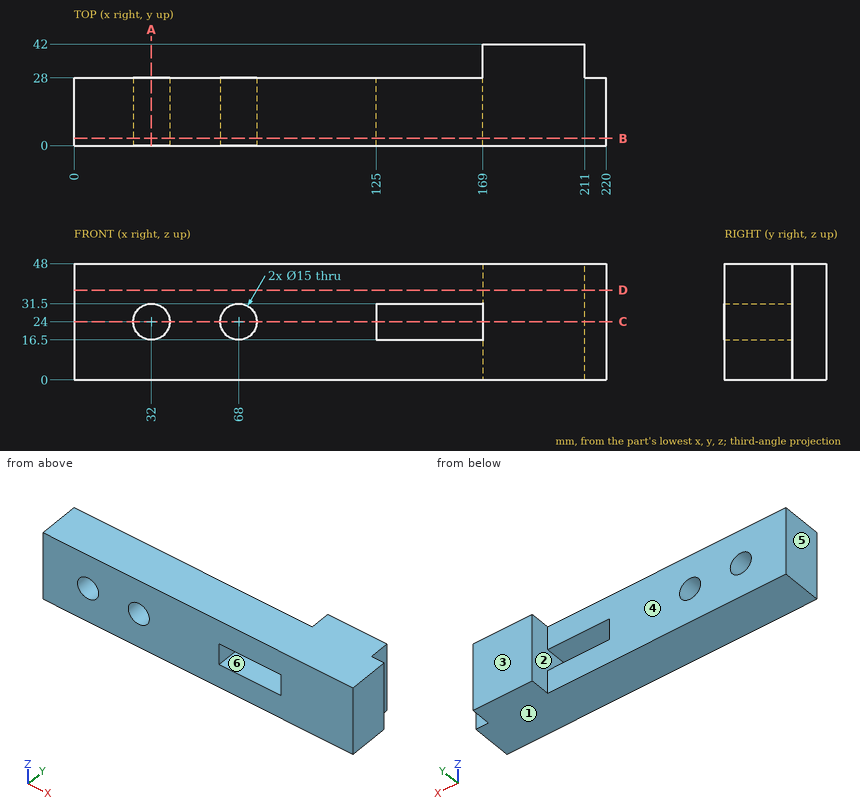
Source: three-view drawing plus pictorial views. Frame: mm from the lowest corner of the part. A direction names the side the tool comes from. Round coordinates to 2 decimals unless told otherwise and drop trailing zeros. Loops run counter-clockwise (first coordinate to the right, second up) from the corner with the lowest first, then second, coordinate; pieces in that order, holes last.
Item 1: Section B-B, the plane y = 3. Output: boundary loops of the cut face in (x, z).
Checked values:
outline: (0, 0) - (220, 0) - (220, 48) - (0, 48) - close; hole circle Ø15 at (32, 24); hole circle Ø15 at (68, 24); hole (125, 16.5) - (169, 16.5) - (169, 31.5) - (125, 31.5) - close
Item 2: Contact query for flat-ended pins moving along their axis: P1, Ø4.5, axis at x = 217, z = 14, coming from the +Y side; P2, Ø8, axis at y = 34.5, z = 12.5, coming from the -X side. Output: stop coordinate, or through.
Checked values:
P1: stops at y = 28
P2: stops at x = 169
Item 3: Section D-D, the plane z = 37. Output: boundary loops of the cut face in (x, y), plus the area to 3 significant figures.
Checked values:
outline: (0, 0) - (220, 0) - (220, 28) - (211, 28) - (211, 42) - (169, 42) - (169, 28) - (0, 28) - close
area: 6,750 mm2
Item 4: Reachability of the marked faces 4, 5 and 6 from +Z, -Z, +X, -X, +Y, -Y: full face, straight path, thin tool, end or side. Return the list, or none.
Checked values:
face 4: +Z, -Z, -X, +Y
face 5: +Z, -Z, -X, +Y, -Y
face 6: +Y, -Y
Item 5: Section C-C, the plane z = 24. Output: boundary loops of the cut face in (x, y).
Checked values:
outline: (0, 0) - (24.5, 0) - (24.5, 28) - (0, 28) - close; (39.5, 0) - (60.5, 0) - (60.5, 28) - (39.5, 28) - close; (75.5, 0) - (125, 0) - (125, 28) - (75.5, 28) - close; (169, 0) - (220, 0) - (220, 28) - (211, 28) - (211, 42) - (169, 42) - close
Item 6: Mould query, pull axis Z, two halves, no side actions, for the marked faces 1, 2 and 3. Classes: released by +Z, released by -Z, zero draft, split by the parting line, or undercut.
Checked values:
face 1: released by -Z
face 2: undercut
face 3: zero draft
Item 7: Section A-A, the plane x = 32. Output: boundary loops of the cut face in (y, z), plus the area to 3 significant figures.
Checked values:
outline: (0, 0) - (28, 0) - (28, 16.5) - (0, 16.5) - close; (0, 31.5) - (28, 31.5) - (28, 48) - (0, 48) - close
area: 924 mm2
Item 8: Line query: L1, parallel to X at y = 18, z = 24.5; L2, parallel to X at y = 19.5, z = 20; L3, parallel to X at y = 38, z = 36.5. Output: solid intervals per line, ascending.
Checked values:
L1: x = 0 to 24.52, 39.48 to 60.52, 75.48 to 125, 169 to 220
L2: x = 0 to 25.66, 38.34 to 61.66, 74.34 to 125, 169 to 220
L3: x = 169 to 211
